Can you work these out from the model? Positions are in its coordinate system, mm. Face numbers are marked on the shaded views. A direction names the side the tool comes from. Give positions to 0.01 mm unless a question says otherwise; leave off trailing zeros. Loops run counter-clockwise (first coordinate to the right, second up) from the corner with the lowest first, then second, coordinate; pieces in that order, holes last. Notation, with made-up numbers: (-17, 55) -> (41, 55) arc R21 cw to (41, 84) -> close; hole circle Ø11 at (14.5, 23). An arc over 180 degrees is marked (long way). Return JSON: item names as keys, results as strings. Group by question number.
Q1. Suppose I cut it at B-B, the plane y = 13. Please give me the cut outline in (x, z), and give its area (3 significant figures).
Q2. Suppose I cut it at C-C, the plane x = 40.5. Please give me the cut outline in (y, z).
Q3. Which directions (+Z, -Z, +X, -X, +Y, -Y) give clear straight access to the entire face, cutting with the end or side of a thin tool? Please do the marked faces 1 and 2.
Q4. Suppose I cut it at A-A, the plane z = 34.5. Please give me the cut outline in (x, y).
Q5. I need wall thicknesses on line 1 along Z through (x, y) = (5.5, 44.5); line 2 along Y through (x, z) = (-15, -33.5). Which ranges of each line are inside material? Lowest first, please. Write a range as [from, to].
Q6. Thinking about a two-plate mould opening in X: for the marked faces 3, 4 and 5, which applies, pulls with the +X half, pulls with the -X half, needs draft (parallel to the pull), parting line crosses it, or undercut?
Q7. Will this pin go through, and if not, where does the flat tip stop? pin 1 (1.5 mm diameter, centred on x = -14.5, z = -9, fed in from -Y).
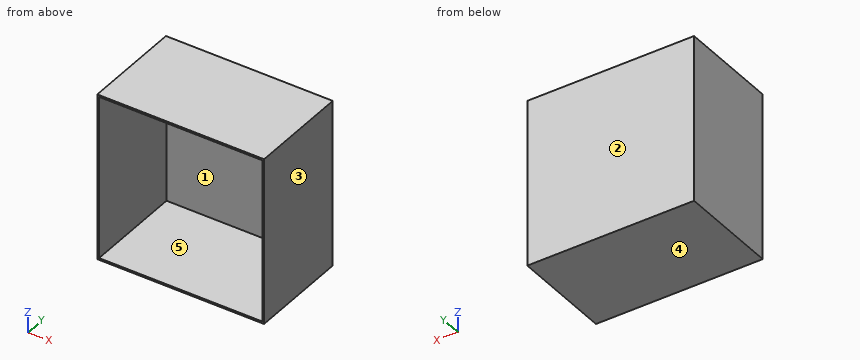
Autodesk Inventor part; units mm, degrees
ref_plane "YZ Plane" through (0, 0, 0) normal (1, 0, 0) x (0, 1, 0)
ref_plane "XZ Plane" through (0, 0, 0) normal (0, 1, 0) x (-1, 0, 0)
ref_plane "XY Plane" through (0, 0, 0) normal (0, 0, 1) x (1, 0, 0)
sketch "Sketch1" plane through (0, 0, 0) normal (0, 1, 0) x (-1, 0, 0)
  line L0 (45, -45) -> (-45, -45)
  line L1 (-45, -45) -> (-45, 45)
  line L2 (-45, 45) -> (45, 45)
  line L3 (45, 45) -> (45, -45)
  line L4 (45, -45) -> (-45, 45) construction
  line L5 (-45, -45) -> (45, 45) construction
  line L6 (-46, -46) -> (46, -46)
  line L7 (46, -46) -> (46, 46)
  line L8 (46, 46) -> (-46, 46)
  line L9 (-46, 46) -> (-46, -46)
  line L10 (-46, -46) -> (46, 46) construction
  line L11 (46, -46) -> (-46, 46) construction
  point P0 (0, 0)
  dimension "d0" = 90
  dimension "d1" = 90
  dimension "d4" = 92
  dimension "d5" = 92
extrude "Extrusion1" add sketch "Sketch1" along normal blind 55
sketch "Sketch2" plane through (0, 55, 0) normal (0, 1, 0) x (1, 0, 0)
  line L0 (-46, 46) -> (-46, -46)
  line L1 (46, 46) -> (-46, 46)
  line L2 (-46, 46) -> (-46, -46)
  line L3 (-46, -46) -> (46, -46)
  line L4 (46, -46) -> (46, 46)
  line L5 (46, 46) -> (-46, -46) construction
  line L6 (-46, 46) -> (46, -46) construction
  point P0 (0, 0)
extrude "Extrusion2" add sketch "Sketch2" along normal blind 1
properties part number "Aluminium block mold"
Ans:
{
 "1": {"outline": "(-46, -46) -> (46, -46) -> (46, 46) -> (-46, 46) -> close; hole (-45, -45) -> (45, -45) -> (45, 45) -> (-45, 45) -> close", "area": "364 mm^2"},
 "2": {"outline": "(0, -46) -> (56, -46) -> (56, 46) -> (0, 46) -> (0, 45) -> (55, 45) -> (55, -45) -> (0, -45) -> close"},
 "3": {"face 1": "-Y", "face 2": "+Z, -Z, +X, -X, +Y"},
 "4": {"outline": "(-46, 0) -> (-45, 0) -> (-45, 55) -> (45, 55) -> (45, 0) -> (46, 0) -> (46, 56) -> (-46, 56) -> close"},
 "5": {"line 1": "z = [-46, -45], [45, 46]", "line 2": "y = [55, 56]"},
 "6": {"face 3": "pulls with the +X half", "face 4": "needs draft", "face 5": "undercut"},
 "7": {"pin 1": "stops at y = 55"}
}
